```python
from build123d import *

# Parameters (mm, degrees)
F0_W         = 609.6
F0_H         = 457.2
F1_DEPTH     = 381
F2_R         = 12.7
F3_T         = -25.4
F4_R         = 209.55
F5_DEPTH     = 25.4
F6_T4_DEPTH  = 165.8906734034
F6_S5_R      = 209.55
F6_T6_DEPTH  = 85
F6_T10_DEPTH = 165.8906734034
F6_S11_R     = 209.55
F6_T12_DEPTH = 85


# Not quite as in the source:
# - a fillet or chamfer that OpenCascade refuses, or shapes differently, is made with other operations: its cross-section is extruded or revolved along the edge and cut away or added


with BuildPart() as f1:
    # F0 (on Top) → F1 (new body)
    with BuildSketch(Plane.XY):
        Rectangle(F0_W, F0_H)
    extrude(amount=F1_DEPTH)

    # F2
    f2_edges = [f1.edges().sort_by_distance(p)[0] for p in [
        (304.8, 0, 381),
        (0, 228.6, 381),
        (-304.8, 0, 381),
        (0, -228.6, 381),
        (-304.8, -228.6, 190.5),
        (304.8, -228.6, 190.5),
        (304.8, 228.6, 190.5),
        (-304.8, 228.6, 190.5),
    ]]
    fillet(f2_edges, radius=F2_R)

    # F3 (hollow: no face is removed)
    offset(amount=F3_T, mode=Mode.SUBTRACT)

    # F4 (on face) → F5 (cut)
    with BuildSketch(Plane.XY.offset(381)):
        Circle(F4_R)
    extrude(amount=-F5_DEPTH, mode=Mode.SUBTRACT)

    # F6: fillet of radius 12.7 on 2 edges, made by hand


with BuildPart() as f6_tool2:
    # F6_s3 → F6_t4 (new body)
    with BuildSketch(Plane.YZ.offset(82.9453367017)):
        with BuildLine():
            ThreePointArc((-215.9, 355.6), (-206.9197438789, 351.8802561211), (-203.2, 342.9))
            Line((-203.2, 342.9), (-203.2, 355.6))
            Line((-203.2, 355.6), (-215.9, 355.6))
        make_face()
    extrude(amount=-F6_T4_DEPTH)

    # F6_s5 → F6_t6 (intersect, symmetric)
    with BuildSketch(Plane.XY.offset(349.3)):
        Circle(F6_S5_R)
    extrude(amount=F6_T6_DEPTH, both=True, mode=Mode.INTERSECT)


with BuildPart() as f1_1:
    add(f1.part)

    # F6_t1: cut F6_tool2
    add(f6_tool2.part, mode=Mode.SUBTRACT)


with BuildPart() as f6_tool8:
    # F6_s9 → F6_t10 (new body)
    with BuildSketch(Plane.YZ.offset(-82.9453367017)):
        with BuildLine():
            ThreePointArc((215.9, 355.6), (206.9197438789, 351.8802561211), (203.2, 342.9))
            Line((203.2, 342.9), (203.2, 355.6))
            Line((203.2, 355.6), (215.9, 355.6))
        make_face()
    extrude(amount=F6_T10_DEPTH)

    # F6_s11 → F6_t12 (intersect, symmetric)
    with BuildSketch(Plane.XY.offset(349.3)):
        Circle(F6_S11_R)
    extrude(amount=F6_T12_DEPTH, both=True, mode=Mode.INTERSECT)


with BuildPart() as f1_2:
    add(f1_1.part)

    # F6_t7: cut F6_tool8
    add(f6_tool8.part, mode=Mode.SUBTRACT)


solid = f1_2.part
```
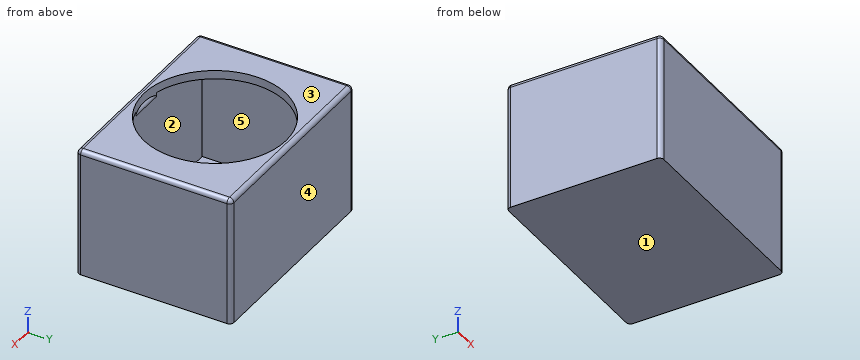
Geometry: final body of the model. Coordinates: model frame, mm. Face numbers are marked on the shaded views. A direction names the side the tool comes from. Coordinates: 2 decimals unless noted, no trailing zeros. Order: outer loops, then holes, each group sorted by start corner. A loop starts at its lowest first (then second) coordinate and runs counter-clockwise, first axis right, second up. Notation, with made-up numbers: (25, 24) -> (29, 24) arc R31 cw to (29, 52) -> close; hole circle Ø4 at (50.25, 65). An arc over 180 degrees is marked (long way). Write item = value, one per line.
(1) Access query for the marked faces 1 and 2. Directions: +Z, -Z, +X, -X, +Y, -Y. A direction counts if a zero-diameter tool reaches every point of the face in a straight line with its end or side. Return the directions, or none.
Solved:
face_1 = -Z, +X, -X, +Y, -Y
face_2 = none
(2) Cut plane B-B on y = 0. Return loops of the section in (x, z).
Solved:
outline = (-304.8, 0) -> (304.8, 0) -> (304.8, 368.3) arc R12.7 ccw to (292.1, 381) -> (209.55, 381) -> (209.55, 355.6) -> (279.4, 355.6) -> (279.4, 25.4) -> (-279.4, 25.4) -> (-279.4, 355.6) -> (-209.55, 355.6) -> (-209.55, 381) -> (-292.1, 381) arc R12.7 ccw to (-304.8, 368.3) -> close
(3) Cut plane C-C on x = 0. Return loops of the section in (y, z).
Solved:
outline = (-228.6, 0) -> (228.6, 0) -> (228.6, 368.3) arc R12.7 ccw to (215.9, 381) -> (209.55, 381) -> (209.55, 353.9) arc R12.7 ccw to (203.2, 342.9) -> (203.2, 25.4) -> (-203.2, 25.4) -> (-203.2, 342.9) arc R12.7 ccw to (-209.55, 353.9) -> (-209.55, 381) -> (-215.9, 381) arc R12.7 ccw to (-228.6, 368.3) -> close
(4) Cut plane A-A on z = 107. Return loops of the section in (x, y), plus the area to 3 significant figures.
Solved:
outline = (-304.8, -215.9) arc R12.7 ccw to (-292.1, -228.6) -> (292.1, -228.6) arc R12.7 ccw to (304.8, -215.9) -> (304.8, 215.9) arc R12.7 ccw to (292.1, 228.6) -> (-292.1, 228.6) arc R12.7 ccw to (-304.8, 215.9) -> close; hole (-279.4, -203.2) -> (279.4, -203.2) -> (279.4, 203.2) -> (-279.4, 203.2) -> close
area = 51,500 mm²
(5) Line query: line 1 (X direction, y = 15, z = 82); line 2 (Y direction, x = 0, z = 357); line 3 (Y direction, x = -184, z = 200). Output: solid intervals per line, ascending.
Solved:
line_1 = -304.8 to -279.4, 279.4 to 304.8
line_2 = -228.6 to -209.55, 209.55 to 228.6
line_3 = -228.6 to -203.2, 203.2 to 228.6
(6) Pull-direction query (Z, two-part tool) for the marked faces 3, 4 and 5; classes: pulls with the +Z half, pulls with the -Z half, needs draft (parallel to the pull), parting line crosses it, or undercut.
Solved:
face_3 = pulls with the +Z half
face_4 = needs draft
face_5 = undercut
